Autodesk Inventor part; units mm, degrees
ref_plane "YZ Plane" through (0, 0, 0) normal (1, 0, 0) x (0, 1, 0)
ref_plane "XZ Plane" through (0, 0, 0) normal (0, 1, 0) x (-1, 0, 0)
ref_plane "XY Plane" through (0, 0, 0) normal (0, 0, 1) x (1, 0, 0)
sketch "Sketch1" plane through (0, 0, 0) normal (0, 0, 1) x (1, 0, 0)
  arc A0 (10.947, -1.0781) -> (10.9857, -0.5614) centre (0, 0) ccw
  circle A1 centre (0, 0) radius 8.75
  line L0 (0, 0) -> (18.5832, 0) construction
  arc A2 (10.9857, -0.5614) -> (8.7477, 0.2024) centre (8.8444, -3.175) ccw
  line L1 (0, 0) -> (16.1968, 0) construction
  line L2 (0, 0) -> (16.1894, 0) construction
  arc A3 (8.6204, -1.5007) -> (10.947, -1.0781) centre (9.2181, 1.8248) ccw
  arc A4 (10.7444, 2.3575) -> (10.6215, 2.8609) centre (0, 0) ccw
  arc A5 (10.6215, 2.8609) -> (8.257, 2.8956) centre (9.3926, -0.2865) ccw
  arc A6 (8.6622, 1.2366) -> (10.7444, 2.3575) centre (8.2031, 4.584) ccw
  arc A7 (9.49, 5.5623) -> (9.2176, 6.003) centre (0, 0) ccw
  arc A8 (9.2176, 6.003) -> (6.958, 5.3055) centre (9.0215, 2.63) ccw
  arc A9 (7.8561, 3.8529) -> (9.49, 5.5623) centre (6.385, 6.8946) ccw
  arc A10 (7.3067, 8.2226) -> (6.9114, 8.5576) centre (0, 0) ccw
  arc A11 (6.9114, 8.5576) -> (4.978, 7.196) centre (7.7672, 5.289) ccw
  arc A12 (6.281, 6.0919) -> (7.3067, 8.2226) centre (3.942, 8.5302) ccw
  arc A13 (4.4082, 10.0781) -> (3.9287, 10.2745) centre (0, 0) ccw
  arc A14 (3.9287, 10.2745) -> (2.5107, 8.3821) centre (5.7527, 7.4304) ccw
  arc A15 (4.0911, 7.7347) -> (4.4082, 10.0781) centre (1.1131, 9.3309) ccw
  arc A16 (1.0781, 10.947) -> (0.5614, 10.9857) centre (0, 0) ccw
  arc A17 (0.5614, 10.9857) -> (-0.2024, 8.7477) centre (3.175, 8.8444) ccw
  arc A18 (1.5007, 8.6204) -> (1.0781, 10.947) centre (-1.8248, 9.2181) ccw
  arc A19 (-2.3575, 10.7444) -> (-2.8609, 10.6215) centre (0, 0) ccw
  arc A20 (-2.8609, 10.6215) -> (-2.8956, 8.257) centre (0.2865, 9.3926) ccw
  arc A21 (-1.2366, 8.6622) -> (-2.3575, 10.7444) centre (-4.584, 8.2031) ccw
  arc A22 (-5.5623, 9.49) -> (-6.003, 9.2176) centre (0, 0) ccw
  arc A23 (-6.003, 9.2176) -> (-5.3055, 6.958) centre (-2.63, 9.0215) ccw
  arc A24 (-3.8529, 7.8561) -> (-5.5623, 9.49) centre (-6.8946, 6.385) ccw
  arc A25 (-8.2226, 7.3067) -> (-8.5576, 6.9114) centre (0, 0) ccw
  arc A26 (-8.5576, 6.9114) -> (-7.196, 4.978) centre (-5.289, 7.7672) ccw
  arc A27 (-6.0919, 6.281) -> (-8.2226, 7.3067) centre (-8.5302, 3.942) ccw
  arc A28 (-10.0781, 4.4082) -> (-10.2745, 3.9287) centre (0, 0) ccw
  arc A29 (-10.2745, 3.9287) -> (-8.3821, 2.5107) centre (-7.4304, 5.7527) ccw
  arc A30 (-7.7347, 4.0911) -> (-10.0781, 4.4082) centre (-9.3309, 1.1131) ccw
  arc A31 (-10.947, 1.0781) -> (-10.9857, 0.5614) centre (0, 0) ccw
  arc A32 (-10.9857, 0.5614) -> (-8.7477, -0.2024) centre (-8.8444, 3.175) ccw
  arc A33 (-8.6204, 1.5007) -> (-10.947, 1.0781) centre (-9.2181, -1.8248) ccw
  arc A34 (-10.7444, -2.3575) -> (-10.6215, -2.8609) centre (0, 0) ccw
  arc A35 (-10.6215, -2.8609) -> (-8.257, -2.8956) centre (-9.3926, 0.2865) ccw
  arc A36 (-8.6622, -1.2366) -> (-10.7444, -2.3575) centre (-8.2031, -4.584) ccw
  arc A37 (-9.49, -5.5623) -> (-9.2176, -6.003) centre (0, 0) ccw
  arc A38 (-9.2176, -6.003) -> (-6.958, -5.3055) centre (-9.0215, -2.63) ccw
  arc A39 (-7.8561, -3.8529) -> (-9.49, -5.5623) centre (-6.385, -6.8946) ccw
  arc A40 (-7.3067, -8.2226) -> (-6.9114, -8.5576) centre (0, 0) ccw
  arc A41 (-6.9114, -8.5576) -> (-4.978, -7.196) centre (-7.7672, -5.289) ccw
  arc A42 (-6.281, -6.0919) -> (-7.3067, -8.2226) centre (-3.942, -8.5302) ccw
  arc A43 (-4.4082, -10.0781) -> (-3.9287, -10.2745) centre (0, 0) ccw
  arc A44 (-3.9287, -10.2745) -> (-2.5107, -8.3821) centre (-5.7527, -7.4304) ccw
  arc A45 (-4.0911, -7.7347) -> (-4.4082, -10.0781) centre (-1.1131, -9.3309) ccw
  arc A46 (-1.0781, -10.947) -> (-0.5614, -10.9857) centre (0, 0) ccw
  arc A47 (-0.5614, -10.9857) -> (0.2024, -8.7477) centre (-3.175, -8.8444) ccw
  arc A48 (-1.5007, -8.6204) -> (-1.0781, -10.947) centre (1.8248, -9.2181) ccw
  arc A49 (2.3575, -10.7444) -> (2.8609, -10.6215) centre (0, 0) ccw
  arc A50 (2.8609, -10.6215) -> (2.8956, -8.257) centre (-0.2865, -9.3926) ccw
  arc A51 (1.2366, -8.6622) -> (2.3575, -10.7444) centre (4.584, -8.2031) ccw
  arc A52 (5.5623, -9.49) -> (6.003, -9.2176) centre (0, 0) ccw
  arc A53 (6.003, -9.2176) -> (5.3055, -6.958) centre (2.63, -9.0215) ccw
  arc A54 (3.8529, -7.8561) -> (5.5623, -9.49) centre (6.8946, -6.385) ccw
  arc A55 (8.2226, -7.3067) -> (8.5576, -6.9114) centre (0, 0) ccw
  arc A56 (8.5576, -6.9114) -> (7.196, -4.978) centre (5.289, -7.7672) ccw
  arc A57 (6.0919, -6.281) -> (8.2226, -7.3067) centre (8.5302, -3.942) ccw
  arc A58 (10.0781, -4.4082) -> (10.2745, -3.9287) centre (0, 0) ccw
  arc A59 (10.2745, -3.9287) -> (8.3821, -2.5107) centre (7.4304, -5.7527) ccw
  arc A60 (7.7347, -4.0911) -> (10.0781, -4.4082) centre (9.3309, -1.1131) ccw
  circle A61 centre (0, 0) radius 2.5
  point P0 (-0.2024, 8.7477)
  point P1 (-1.2366, 8.6622)
  point P2 (-2.8956, 8.257)
  point P3 (-3.8529, 7.8561)
  point P4 (-5.3055, 6.958)
  point P5 (-8.7477, -0.2024)
  point P6 (-8.257, -2.8956)
  point P7 (-7.8561, -3.8529)
  point P8 (-6.958, -5.3055)
  point P9 (-4.0911, -7.7347)
  point P10 (-2.5107, -8.3821)
  point P11 (0.2024, -8.7477)
  point P12 (1.2366, -8.6622)
  point P13 (2.8956, -8.257)
  point P14 (3.8529, -7.8561)
  point P15 (7.196, -4.978)
  point P16 (7.7347, -4.0911)
  point P17 (8.3821, -2.5107)
  point P18 (8.6622, 1.2366)
  point P19 (8.257, 2.8956)
  point P20 (7.8561, 3.8529)
  point P21 (6.958, 5.3055)
  point P22 (4.978, 7.196)
  point P23 (4.0911, 7.7347)
  point P24 (2.5107, 8.3821)
  dimension "d2" = 17.5
  dimension "d1" = 22
  dimension "d8" = 360
  dimension "d10" = 5
extrude "Extrusion1" add sketch "Sketch1" along normal blind 10
properties part number "PLANETARIO SOL"
The model under review builds one solid part; all positions refer to its coordinate system, in mm. A direction names the side the tool comes from. Round coordinates to 2 decimals unless told otherwise and drop trailing zeros. Answer as a JSON object with one key per item and string values.
Item 1: Clearance check with flat-ended pins moving along their axes: P1, Ø1.5, axis at x = 8, z = 7.5, coming from the -Y side; P2, Ø5, axis at x = 6, z = 5.5, coming from the +Y side; P3, Ø3, axis at x = 3, z = 7.5, coming from the -Y side. State where each tip first meets the part, or that it passes through.
Check sheet entries:
{"P1": "y = -7.31", "P2": "y = 10.27", "P3": "y = -10.74"}
Item 2: Tool access review of faces 1 (the face through (1.617, -9.819, 4.93)), 2 (the face through (-8.042, 5.808, 4.93)), 3 (the face through (3.387, -8.068, 4.93)), 4 (the face through (9.819, 1.617, 4.93)), 5 (the face through (-3, 0, 10)): name each direction out of +Z, -Z, +X, -X, +Y, -Y from which nothing blocks a thin tool from reaching the whole face with its end or side.
Check sheet entries:
{"face 1": "+Z, -Z, -Y", "face 2": "+Z, -Z, -X", "face 3": "+Z, -Z", "face 4": "+Z, -Z, +X", "face 5": "+Z, +X, -X, +Y, -Y"}
Item 3: The part is to be moulded in two halves that separate along X. For faces 6 (the face through (-8.068, -3.387, 4.93)), 7 (the face through (9.443, -3.039, 4.93)), 8 (the face through (-8.72, -0.73, 4.93)), 9 (the face through (1.497, 9.839, 4.93)), say which applies: +X half, -X half, draft (parallel to the pull), parting line (faces both ways), or undercut.
Check sheet entries:
{"face 6": "undercut", "face 7": "+X half", "face 8": "-X half", "face 9": "undercut"}
Item 4: For line 1 along X through (y, z) = (-8, 4); line 2 along Y through (x, z) = (-1.75, 4.5); line 3 along Y through (x, z) = (-0.75, 3), list the stretches that pass through material, from the lowest coordinate up.
Check sheet entries:
{"line 1": "-7.28 to -5.75, -4.22 to 3.54, 3.93 to 5.85", "line 2": "-8.57 to -1.79, 1.79 to 10.04", "line 3": "-10.97 to -2.38, 2.38 to 8.72"}
